```python
from build123d import *

# Parameters (mm, degrees)
F0_W     = 101.6
F0_H     = 127
F1_DEPTH = 76.2
F2_T     = -3.81
F3_R     = 30
F4_R     = 2.5
F5_DEPTH = 76.2


with BuildPart() as f1:
    # F0 (on Top) → F1 (new body)
    with BuildSketch(Plane.XY):
        Rectangle(F0_W, F0_H)
    extrude(amount=F1_DEPTH)

    # F2
    f2_openings = [f1.faces().sort_by_distance(p)[0] for p in [
        (0, 0, 76.2),
    ]]
    offset(amount=F2_T, openings=f2_openings)

    # F3
    f3_edges = [f1.edges().sort_by_distance(p)[0] for p in [
        (0, 59.69, 3.81),
        (0, -59.69, 3.81),
    ]]
    fillet(f3_edges, radius=F3_R)

    # F4
    f4_edges = [f1.edges().sort_by_distance(p)[0] for p in [
        (-46.99, -50.903203, 12.596797),
        (46.99, -50.903203, 12.596797),
    ]]
    fillet(f4_edges, radius=F4_R)

    # F5 (add): a face of the model
    f5_faces = [f1.faces().sort_by_distance(p)[0] for p in [
        (0, -61.3163935563, 76.2),
    ]]
    extrude(f5_faces, amount=-F5_DEPTH)


solid = f1.part
```
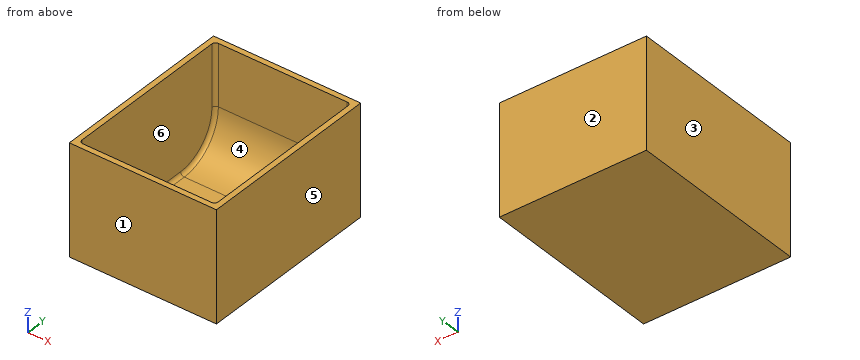
Geometry: final body of the model. Coordinates: model frame, mm. Face numbers are marked on the shaded views. A direction names the side the tool comes from. Round coordinates to 2 decimals unless told otherwise and drop trailing zeros. Order: outer loops, then holes, each group sorted by start corner. A loop starts at its lowest first (then second) coordinate and runs counter-clockwise, first axis right, second up. Notation, with made-up numbers: (49, -21.5) - (101, -21.5) arc R24 cw to (101, 6.5) - close; hole circle Ø3 at (-28, 39). An arc over 180 degrees is marked (long way). Use CSV: the item, a comma, the result in double quotes. Start each with the question number.
Q1. Section query B-B (x = -29.5). Return loops of the section in (y, z).
Q2. Section query C-C (y = -15). Return loops of the section in (x, z).
Q3. Mould query, pull axis Y, two halves, no side actions, for the marked faces 1, 2, 3 and 4. Classes: +Y half, -Y half, draft (parallel to the pull), parting line (faces both ways), or undercut.
Q4. Access query for the marked faces 5 and 6. Directions: +Z, -Z, +X, -X, +Y, -Y. A direction counts if a zero-diameter tool reaches every point of the face in a straight line with its end or side. Return the directions, or none.
Q5. First-contact query: pin 1 (5 mm diameter, centred on x = -37, y = 0, fed in from +Z). Flat tip, straight axial feed; report the tip coordinate or a pass-through.
Q6. Material intervals for line 1 along X through (y, z) = (55, 69); line 2 along Y through (x, z) = (-39, 56.5); line 3 along Z through (x, y) = (-43, 6), sorted ascending. Write a range as from..to.
Q7. Section query A-A (z = 61). Return loops of the section in (x, y).
Result set:
1,outline,"(-63.5, 0) - (63.5, 0) - (63.5, 76.2) - (59.69, 76.2) - (59.69, 33.81) arc R30 cw to (29.69, 3.81) - (-29.69, 3.81) arc R30 cw to (-59.69, 33.81) - (-59.69, 76.2) - (-63.5, 76.2) - close"
2,outline,"(-50.8, 0) - (50.8, 0) - (50.8, 76.2) - (46.99, 76.2) - (46.99, 6.31) arc R2.5 cw to (44.49, 3.81) - (-44.49, 3.81) arc R2.5 cw to (-46.99, 6.31) - (-46.99, 76.2) - (-50.8, 76.2) - close"
3,face 1,"-Y half"
3,face 2,"+Y half"
3,face 3,"draft"
3,face 4,"undercut"
4,face 5,"+Z, -Z, +X, +Y, -Y"
4,face 6,"+Z"
5,pin 1,"stops at z = 3.81"
6,line 1,"x = -50.8..-46.99, 46.99..50.8"
6,line 2,"y = -63.5..-59.69, 59.69..63.5"
6,line 3,"z = 0..3.81"
7,outline,"(-50.8, -63.5) - (50.8, -63.5) - (50.8, 63.5) - (-50.8, 63.5) - close; hole (-46.99, -57.19) arc R2.5 ccw to (-44.49, -59.69) - (44.49, -59.69) arc R2.5 ccw to (46.99, -57.19) - (46.99, 57.19) arc R2.5 ccw to (44.49, 59.69) - (-44.49, 59.69) arc R2.5 ccw to (-46.99, 57.19) - close"
